Verification items for the finished model (mm, model axes). A direction names the side the tool comes from. Round coordinates to 2 decimals unless told otherwise and drop trailing zeros. Order: outer loops, then holes, each group sorted by start corner. A loop starts at its lowest first (then second) coordinate and runs counter-clockwise, first axis right, second up. Notation, with made-up numbers: M 48.5,17.25 L 74.5,17.25 A10 ccw 74.5,25.25 Z; hole C 35.25,40.5 d9. An arc over 180 degrees is marked long. Use one line per item in the form item = value. Start each with the question number.
Item 1: Tool access check on faces 1 (the flat face through (-5, -229, 0)), 2 (the flat face through (-10, 193, 0)), 3 (the flat face through (5, -229, 0)). Record the directions out of +Z, -Z, +X, -X, +Y, -Y that give a thin tool (end or side, any length) a straight path to the whole face; none if there is none.
Item 2: Release check for a two-part mould opening along Y. For faces 4 (the cylindrical face through (0.07, -228.143, 3.252)), 5 (the flat face through (20, 213.4, -15.2)), 6 (the cylindrical face through (-10.703, -179.514, -0.414)) record: +Y half, -Y half, draft (parallel to the pull), parting line (faces both ways), or undercut.
Item 3: Thickness scan on probe 1 along Y at (x, z) = (1, 0); probe 2 along X at (y, z) = (-215, -21.5); probe 3 along X at (y, z) = (-14.5, -1.5). Record the ranges inside material, lowest first. Write a range as [from, to].
Item 4: Cross-section at A-A on y = 213.5. Enter the section's corners in (x, z).
Item 5: Cross-section at B-B on x = 0. Enter the section's corners in (y, z), then the cut area to 3 significant figures.
Item 6: Cross-section at C-C on y = -21.5. Enter the section's corners in (x, z).
Item 7: Go/stop test with flat-tipped pins: pin 1 Ø4 at (x, z) = (27.5, 6.5) entering from -Y; pin 2 Ø10 at (x, z) = (-1, -9.5) entering from +Y; pin 3 Ø1 at (y, z) = (-78.5, 9.5) entering from +X. Record where each tip stops, or that it passes through.
from build123d import *

# Parameters (mm, degrees)
SKETCH1_R               = 30
BOSS_EXTRUDE1_DEPTH     = 243.5
CUT_EXTRUDE1_DEPTH      = 70
FILLET1_R               = 9
FILLET2_R               = 9
SKETCH4_R               = 15
CUT_EXTRUDE2_DEPTH      = 70
CUT_EXTRUDE3_DEPTH      = 70
CUT_EXTRUDE3_DEPTH_BACK = 70
CUT_EXTRUDE4_START      = -70
CUT_EXTRUDE4_DEPTH      = 70
SKETCH8_R               = 15
CUT_EXTRUDE5_DEPTH      = 60
CUT_EXTRUDE8_DEPTH      = 60
CUT_EXTRUDE8_DEPTH_BACK = 60
FILLET3_R               = 20
FILLET4_R               = 20


with BuildPart() as part:
    # Sketch1 → Boss-Extrude1 (new, symmetric)
    with BuildSketch(Plane(origin=(0, 0, 0), x_dir=(1, 0, 0), z_dir=(0, 1, 0))):
        with Locations(Location((0, 0, 0), (0, 0, 270))):
            Circle(SKETCH1_R)
    extrude(amount=BOSS_EXTRUDE1_DEPTH, both=True)

    # Sketch3 → Cut-Extrude1 (cut)
    with BuildSketch(Plane(origin=(0, 243.5, 0), x_dir=(1, 0, 0), z_dir=(0, 1, 0))):
        with BuildLine():
            Line((-10, 28.284271247), (-10, -28.284271247))
            ThreePointArc((-10, -28.284271247), (0, -30), (10, -28.284271247))
            Line((10, -28.284271247), (10, 28.284271247))
            ThreePointArc((10, 28.284271247), (0, 30), (-10, 28.284271247))
        make_face()
        with BuildLine():
            Line((-20, 22.360679775), (-20, -22.360679775))
            ThreePointArc((-20, -22.360679775), (-30, 0), (-20, 22.360679775))
        make_face()
        with BuildLine():
            Line((20, 22.360679775), (20, -22.360679775))
            ThreePointArc((20, -22.360679775), (30, 0), (20, 22.360679775))
        make_face()
    extrude(amount=-CUT_EXTRUDE1_DEPTH, mode=Mode.SUBTRACT)

    # Fillet1
    fillet1_edges = [part.edges().sort_by_distance(p)[0] for p in [
        (-20, 173.5, 0),
    ]]
    fillet(fillet1_edges, radius=FILLET1_R)

    # Fillet2
    fillet2_edges = [part.edges().sort_by_distance(p)[0] for p in [
        (20, 173.5, 0),
    ]]
    fillet(fillet2_edges, radius=FILLET2_R)

    # Sketch4 → Cut-Extrude2 (cut)
    with BuildSketch(Plane(origin=(20, 0, 0), x_dir=(0, 0, -1), z_dir=(1, 0, 0))):
        with Locations((0, 213.5)):
            Circle(SKETCH4_R)
    extrude(amount=-CUT_EXTRUDE2_DEPTH, mode=Mode.SUBTRACT)

    # Sketch6 → Cut-Extrude3 (cut, two sides: drawn at the far end of the back side and taken through both)
    with BuildSketch(Plane(origin=(0, 0, 0), x_dir=(0, 0, -1), z_dir=(1, 0, 0)).offset(-CUT_EXTRUDE3_DEPTH_BACK)):
        with BuildLine():
            Line((-1.96e-07, 243.5), (-28.284271247, 243.5))
            Line((-28.284271247, 243.5), (-28.284271247, 223.5))
            ThreePointArc((-28.284271247, 223.5), (-17.320508156, 237.994897371), (-1.96e-07, 243.5))
        make_face()
        with BuildLine():
            Line((28.284271247, 243.5), (-1.96e-07, 243.5))
            ThreePointArc((-1.96e-07, 243.5), (17.320507996, 237.994897484), (28.284271247, 223.5))
            Line((28.284271247, 223.5), (28.284271247, 243.5))
        make_face()
    extrude(amount=CUT_EXTRUDE3_DEPTH + CUT_EXTRUDE3_DEPTH_BACK, mode=Mode.SUBTRACT)

    # Sketch7 → Cut-Extrude4 (cut)
    with BuildSketch(Plane.XZ.offset(243.5).offset(CUT_EXTRUDE4_START)):
        with BuildLine():
            Line((-5, 29.580398915), (-5, -29.580398915))
            ThreePointArc((-5, -29.580398915), (-30, 0), (-5, 29.580398915))
        make_face()
        with BuildLine():
            Line((5, 29.580398915), (5, -29.580398915))
            ThreePointArc((5, -29.580398915), (30, 0), (5, 29.580398915))
        make_face()
    extrude(amount=CUT_EXTRUDE4_DEPTH, mode=Mode.SUBTRACT)

    # Sketch8 → Cut-Extrude5 (cut)
    with BuildSketch(Plane(origin=(5, 0, 0), x_dir=(0, 0, -1), z_dir=(1, 0, 0))):
        with Locations((0, -213.5)):
            Circle(SKETCH8_R)
    extrude(amount=-CUT_EXTRUDE5_DEPTH, mode=Mode.SUBTRACT)

    # Sketch10 → Cut-Extrude8 (cut, two sides: drawn at the far end of the back side and taken through both)
    with BuildSketch(Plane(origin=(0, 0, 0), x_dir=(0, 0, -1), z_dir=(1, 0, 0)).offset(-CUT_EXTRUDE8_DEPTH_BACK)):
        with BuildLine():
            Line((30, -243.5), (30, -213.5))
            ThreePointArc((30, -213.5), (21.213203436, -234.713203436), (0, -243.5))
            Line((0, -243.5), (30, -243.5))
        make_face()
        with BuildLine():
            ThreePointArc((0, -243.5), (-21.213203436, -234.713203436), (-30, -213.5))
            Line((-30, -213.5), (-30, -243.5))
            Line((-30, -243.5), (0, -243.5))
        make_face()
    extrude(amount=CUT_EXTRUDE8_DEPTH + CUT_EXTRUDE8_DEPTH_BACK, mode=Mode.SUBTRACT)

    # Fillet3
    fillet3_edges = [part.edges().sort_by_distance(p)[0] for p in [
        (5, -173.5, 0),
    ]]
    fillet(fillet3_edges, radius=FILLET3_R)

    # Fillet4
    fillet4_edges = [part.edges().sort_by_distance(p)[0] for p in [
        (-5, -173.5, 0),
    ]]
    fillet(fillet4_edges, radius=FILLET4_R)


solid = part.part
Output values:
q1.face_1 = +Z, -Z, -X, -Y
q1.face_2 = +Z, -Z, +Y
q1.face_3 = +Z, -Z, +X, -Y
q2.face_4 = undercut
q2.face_5 = draft
q2.face_6 = -Y half
q3.probe_1 = [-243.5, -228.5], [-198.5, 173.5]
q3.probe_2 = [-5, 5]
q3.probe_3 = [-29.96, 29.96]
q4.outline = M -20,-22.36 A30 ccw -10,-28.28 L -10,-15 L -20,-15 Z; M -20,15 L -10,15 L -10,28.28 A30 ccw -20,22.36 Z; M 10,-28.28 A30 ccw 20,-22.36 L 20,-15 L 10,-15 Z; M 10,15 L 20,15 L 20,22.36 A30 ccw 10,28.28 Z
q5.outline = M -213.5,-30 L 173.5,-30 L 173.5,30 L -213.5,30 A30 ccw Z; hole C -213.5,0 d30
q5.area = 23,900 mm2
q6.outline = C 0,0 d60
q7.pin_1 = -173.5
q7.pin_2 = 173.5
q7.pin_3 = 28.62
